Geometry: see drawing. Coordinates: mm, zero at the bounding-box minimum. A direction names the side the tool comes from. Round coordinates to 2 decimals unless told otherwise and drop trailing zeros. Loops run counter-clockwise (first coordinate to the right, second up) from the corner with the lowest first, then second, coordinate; pieces in that order, holes last.
(1) Section D-D, the plane z = 29. Return the cut outline in (x, y).
(2) Section A-A, the plane x = 15.25. Return the cut outline in (y, z).
(3) Mould query, pull axis Z, two halves, no side actions, for the marked faces 3 and 4. Classes: pulls with the +Z half, pulls with the -Z half, needs draft (parallel to the pull), parting line crosses it, or undercut.
(4) First-contact query: pin 1 Ø0.5 at (y, z) = (11, 11.5) entering from -X; pin 2 Ø1.3 at (x, z) = (15.25, 2) entering from +Y; pin 3 Ø0.5 at (y, z) = (11.5, 17.5) entering from +X; pin 4 Ø5 at (x, z) = (13.5, 15) entering from -Y. Flat tips, straight axial feed; report the tip coordinate or a pass-through.
(5) Material intervals for probe 1 along Z at (x, y) = (15.25, 9.7); probe 2 along X at (y, z) = (11.25, 24); probe 3 along Z at (x, y) = (9.5, 1.5), sorted ascending.
(6) Section B-B, the plane y = 3.5. Return the cut outline in (x, z).
(7) Set-up query: the marked faces 1 and 2. Return all of +Z, -Z, +X, -X, +Y, -Y with unobstructed straight access to the full face (end or side cutting, diameter ignored); none if empty.
(8) Section C-C, the plane z = 18. Return the cut outline in (x, y), plus the area to 3 significant figures.
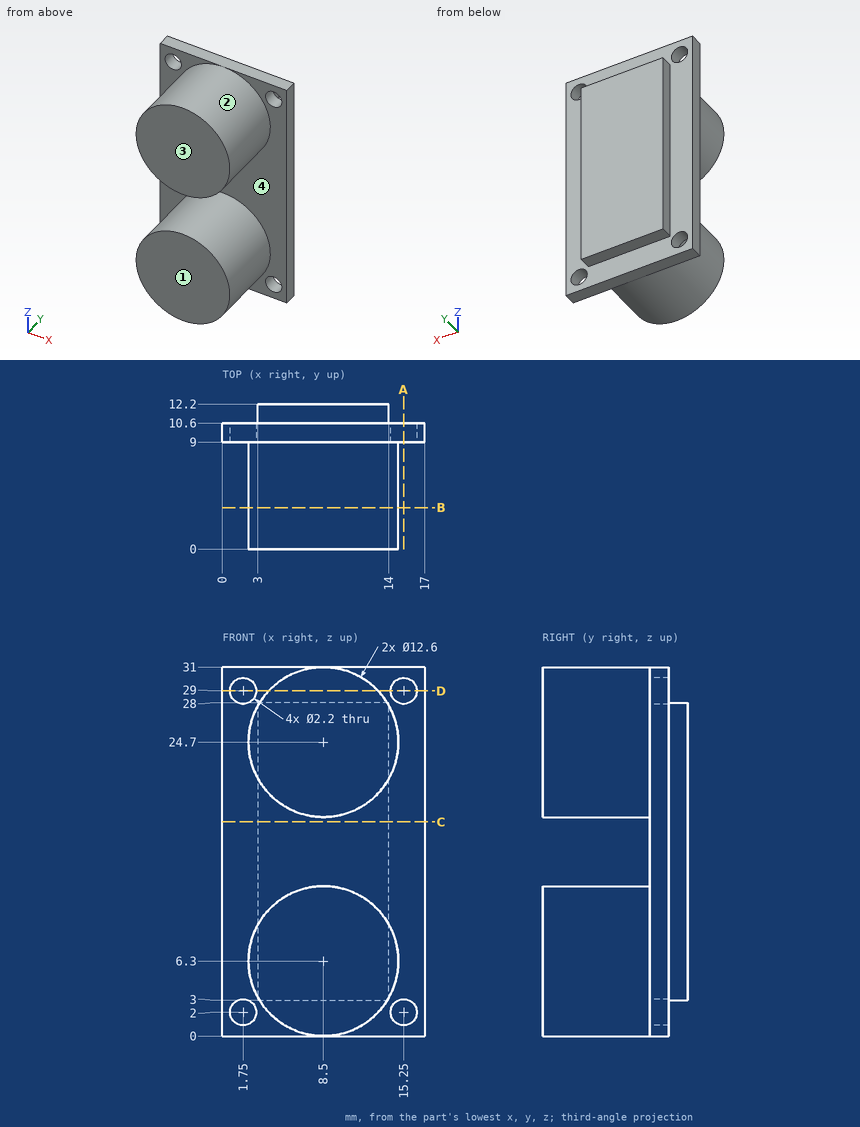
Output values:
1. outline: (0, 9) - (0.65, 9) - (0.65, 10.6) - (0, 10.6) - close; (2.85, 9) - (3.9, 9) - (3.9, 0) - (13.1, 0) - (13.1, 9) - (14.15, 9) - (14.15, 10.6) - (2.85, 10.6) - close; (16.35, 9) - (17, 9) - (17, 10.6) - (16.35, 10.6) - close
2. outline: (9, 0) - (10.6, 0) - (10.6, 0.9) - (9, 0.9) - close; (9, 3.1) - (10.6, 3.1) - (10.6, 27.9) - (9, 27.9) - close; (9, 30.1) - (10.6, 30.1) - (10.6, 31) - (9, 31) - close
3. face 3: needs draft
3. face 4: undercut
4. pin 1: stops at x = 3
4. pin 2: passes through
4. pin 3: stops at x = 14
4. pin 4: stops at y = 9
5. probe 1: z = 0 to 0.9, 3.1 to 27.9, 30.1 to 31
5. probe 2: x = 3 to 14
5. probe 3: z = 0.08 to 12.52, 18.48 to 30.92
6. outline: circle Ø12.6 at (8.5, 6.3); circle Ø12.6 at (8.5, 24.7)
7. face 1: +Z, -Z, +X, -X, -Y
7. face 2: -Y
8. outline: (0, 9) - (17, 9) - (17, 10.6) - (14, 10.6) - (14, 12.2) - (3, 12.2) - (3, 10.6) - (0, 10.6) - close
8. area: 44.8 mm2
